Part model, mm, in its own coordinate system. A direction names the side the tool comes from. Give positions to 0.01 mm unless a question says otherwise; leave off trailing zeros. Order: outer loops, then holes, each group sorted by start corner. A loop starts at its lowest first (then second) coordinate and runs counter-clockwise, first axis right, second up. Notation, with made-up numbers: M 32.25,-26.5 L 83.25,-26.5 A20 ccw 83.25,-7.5 Z; hole C 88.25,-11.5 d8. An arc over 180 degrees is marked long. Return JSON: item names as keys, results as strings.
from build123d import *

# Parameters (mm, degrees)
BOSS_EXTRU_1_DEPTH      = 97.5
BOSS_EXTRU_1_DEPTH_BACK = 97.5
ESQUISSE1_W             = 12.5
ESQUISSE1_H             = 25.4
ENL_V_MAT_EXTRU_1_DEPTH = 102.526646749
CONG_1_R                = 10
CONG_2_R                = 10
CONG_3_R                = 10
CONG_4_R                = 10
BOSS_EXTRU_4_DEPTH      = 12.5
ENL_V_MAT_EXTRU_2_DEPTH = 102.526646749


with BuildPart() as part:
    # Esquisse1 → Boss.-Extru.1 (new, two sides: drawn at the far end of the back side and taken through both)
    with BuildSketch(Plane.XY.offset(-BOSS_EXTRU_1_DEPTH_BACK)):
        with Locations((6.25, 12.7)):
            Rectangle(ESQUISSE1_W, ESQUISSE1_H)
    extrude(amount=BOSS_EXTRU_1_DEPTH + BOSS_EXTRU_1_DEPTH_BACK)

    # Esquisse3 → Enlèv. mat.-Extru.1 (cut, through all)
    with BuildSketch(Plane.ZY):
        with BuildLine():
            Line((25.4, 16.765), (87.5, 16.765))
            ThreePointArc((87.5, 16.765), (91.565, 12.7), (87.5, 8.635))
            Line((87.5, 8.635), (25.4, 8.635))
            ThreePointArc((25.4, 8.635), (21.335, 12.7), (25.4, 16.765))
        make_face()
    enl_v_mat_extru_1 = extrude(amount=-ENL_V_MAT_EXTRU_1_DEPTH, mode=Mode.SUBTRACT)

    # Symétrie1: Enlèv. mat.-Extru.1 across plane
    add(enl_v_mat_extru_1.mirror(Plane.XY), mode=Mode.SUBTRACT)

    # Congé1
    cong_1_edges = [part.edges().sort_by_distance(p)[0] for p in [
        (6.25, 0, -97.5),
    ]]
    fillet(cong_1_edges, radius=CONG_1_R)

    # Congé2
    cong_2_edges = [part.edges().sort_by_distance(p)[0] for p in [
        (6.25, 25.4, -97.5),
    ]]
    fillet(cong_2_edges, radius=CONG_2_R)

    # Congé3
    cong_3_edges = [part.edges().sort_by_distance(p)[0] for p in [
        (6.25, 0, 97.5),
    ]]
    fillet(cong_3_edges, radius=CONG_3_R)

    # Congé4
    cong_4_edges = [part.edges().sort_by_distance(p)[0] for p in [
        (6.25, 25.4, 97.5),
    ]]
    fillet(cong_4_edges, radius=CONG_4_R)

    # Esquisse4 → Boss.-Extru.4 (add)
    with BuildSketch(Plane(origin=(12.5, 0, 0), x_dir=(0, 0, -1), z_dir=(1, 0, 0))):
        Polygon((0, 0), (-56.566309771, 0), (-86.246950766, 0), (-76, -16), (0, -16), (76, -16), (86.246950766, 0), (56.566309771, 0), align=None)
    extrude(amount=-BOSS_EXTRU_4_DEPTH)

    # Esquisse5 → Enlèv. mat.-Extru.2 (cut, through all)
    with BuildSketch(Plane(origin=(12.5, 0, 0), x_dir=(0, 0, -1), z_dir=(1, 0, 0))):
        with BuildLine():
            Line((-62.01, -0.935), (-37, -0.935))
            ThreePointArc((-37, -0.935), (-32.935, -5), (-37, -9.065))
            Line((-37, -9.065), (-62.01, -9.065))
            ThreePointArc((-62.01, -9.065), (-66.075, -5), (-62.01, -0.935))
        make_face()
    enl_v_mat_extru_2 = extrude(amount=-ENL_V_MAT_EXTRU_2_DEPTH, mode=Mode.SUBTRACT)

    # Symétrie2: Enlèv. mat.-Extru.2 across plane
    add(enl_v_mat_extru_2.mirror(Plane.XY), mode=Mode.SUBTRACT)


solid = part.part
Q1. Band-saw the part on A-A (z = -60). Give the cut face in (x, y) (3 decimals).
Established:
{"outline": "M 0,-16 L 12.5,-16 L 12.5,-9.065 L 0,-9.065 Z; M 0,-0.935 L 12.5,-0.935 L 12.5,8.635 L 0,8.635 Z; M 0,16.765 L 12.5,16.765 L 12.5,25.4 L 0,25.4 Z"}
Q2. Band-saw the part on B-B (y = 12.7). Give the cut face in (x, z) (3 decimals).
Established:
{"outline": "M 0,-97.5 L 12.5,-97.5 L 12.5,-91.565 L 0,-91.565 Z; M 0,-21.335 L 12.5,-21.335 L 12.5,21.335 L 0,21.335 Z; M 0,91.565 L 12.5,91.565 L 12.5,97.5 L 0,97.5 Z"}
Q3. Two-plate mould, pull along Z, no slides. Class faces 1 (the flat face through (6.338, -8.112, -81.052)), 2 (the cylindrical face through (6.162, 12.789, -91.564)), 3 (the cylindrical face through (6.34, 22.39, 94.65)): +Z half, -Z half, draft (parallel to the pull), parting line (faces both ways), or undercut.
Established:
{"face 1": "-Z half", "face 2": "undercut", "face 3": "+Z half"}
Q4. Band-saw the part on C-C (x = 6). Give the cut face in (y, z) (3 decimals).
Established:
{"outline": "M -16,-76 L 0,-86.247 L 0,-87.5 A10 ccw 10,-97.5 L 15.4,-97.5 A10 ccw 25.4,-87.5 L 25.4,87.5 A10 ccw 15.4,97.5 L 10,97.5 A10 ccw 0,87.5 L 0,86.247 L -16,76 Z; hole M -9.065,-62.01 A4.065 ccw -0.935,-62.01 L -0.935,-37 A4.065 ccw -9.065,-37 Z; hole M -9.065,37 A4.065 ccw -0.935,37 L -0.935,62.01 A4.065 ccw -9.065,62.01 Z; hole M 8.635,-87.5 A4.065 ccw 16.765,-87.5 L 16.765,-25.4 A4.065 ccw 8.635,-25.4 Z; hole M 8.635,25.4 A4.065 ccw 16.765,25.4 L 16.765,87.5 A4.065 ccw 8.635,87.5 Z"}
Q5. 3-axis set-ups, long thin cutter, end or side, ignore diameter. For faces 4 (the cylindrical face through (6.34, 2.85, -94.49)), 5 (the flat face through (6, -9.065, -49)): which of +Z, -Z, +X, -X, +Y, -Y reach the whole face in a straight line?
Established:
{"face 4": "-Z, +X, -X, -Y", "face 5": "+X, -X"}
Q6. Probe line 1 along Z through (x, y) = (6.5, 13); line 2 along Y through (x, z) = (8.5, 55.5) (3 decimals); line 3 along Y through (x, z) = (3.25, -26.5) (3 decimals). List the from-to ranges inside material, lowest first.
Established:
{"line 1": "z = -97.5 to -91.55, -21.35 to 21.35, 91.55 to 97.5", "line 2": "y = -16 to -9.065, -0.935 to 8.635, 16.765 to 25.4", "line 3": "y = -16 to 8.635, 16.765 to 25.4"}
Q7. Band-saw the part on D-D (z = 78). Give the cut face in (x, y) (3 decimals).
Established:
{"outline": "M 0,-12.877 L 12.5,-12.877 L 12.5,8.635 L 0,8.635 Z; M 0,16.765 L 12.5,16.765 L 12.5,25.4 L 0,25.4 Z"}
Q8. Pin check, flat tips, straight feed: pin 1 (3 mm diameter, centred on x = 11, y = 1, fed in from -Z); pin 2 (0.6 mm diameter, centred on x = 5.5, z = 87, fed in from -Y); pin 3 (2 mm diameter, centred on x = 4.5, y = -9, fed in from -Z). Stop position of each tip, or through.
Established:
{"pin 1": "stops at z = -94.11", "pin 2": "stops at y = 0", "pin 3": "stops at z = -81.12"}
